Could you check a few things on this drawing? It's one solid part, dimensions in mm from its lowest x, y, z. A direction names the side the tool comes from. Give positions to 0.01 mm unless a question says otherwise; leave off trailing zeros. Order: outer loops, then holes, each group sorted by start corner. A loop starts at its lowest first (then second) coordinate and runs counter-clockwise, first axis right, second up.
Item 1: If we mould it in two halves opening along Z, with no side actions, what happens to the marked faces 1, 2, 3 and 4? For each: +Z half, -Z half, draft (parallel to the pull), parting line (faces both ways), or undercut.
Item 2: I want a section at A-A, the plane z = 14. Write out the boundary of the cut face in (x, y), then the cut area to 3 significant figures.
Item 3: I want a section at C-C, the plane y = 15. Write out the boundary of the cut face in (x, z), then the cut area to 3 significant figures.
Item 4: Which directions (+Z, -Z, +X, -X, +Y, -Y) give clear straight access to the entire face, cutting with the end or side of a thin tool? Please do the marked faces 5 and 6.
Item 5: I'm going to push flat-ended pins straight in: pin 1 Ø6 at (x, y) = (50.5, 20.5) entering from -Z; pin 2 Ø5 at (x, z) = (73, 67) entering from +Y. Where does each tip first touch, or does it pass through?
Item 6: If I drill on line 1 along X through (y, z) = (25, 46); line 2 along Z through (x, y) = (40.5, 5.5), over which ranges is the centre line in solid material (lowest first)?
Item 7: I want a section at B-B, the plane x = 15. Write out the boundary of the cut face in (y, z), then the cut area to 3 significant figures.
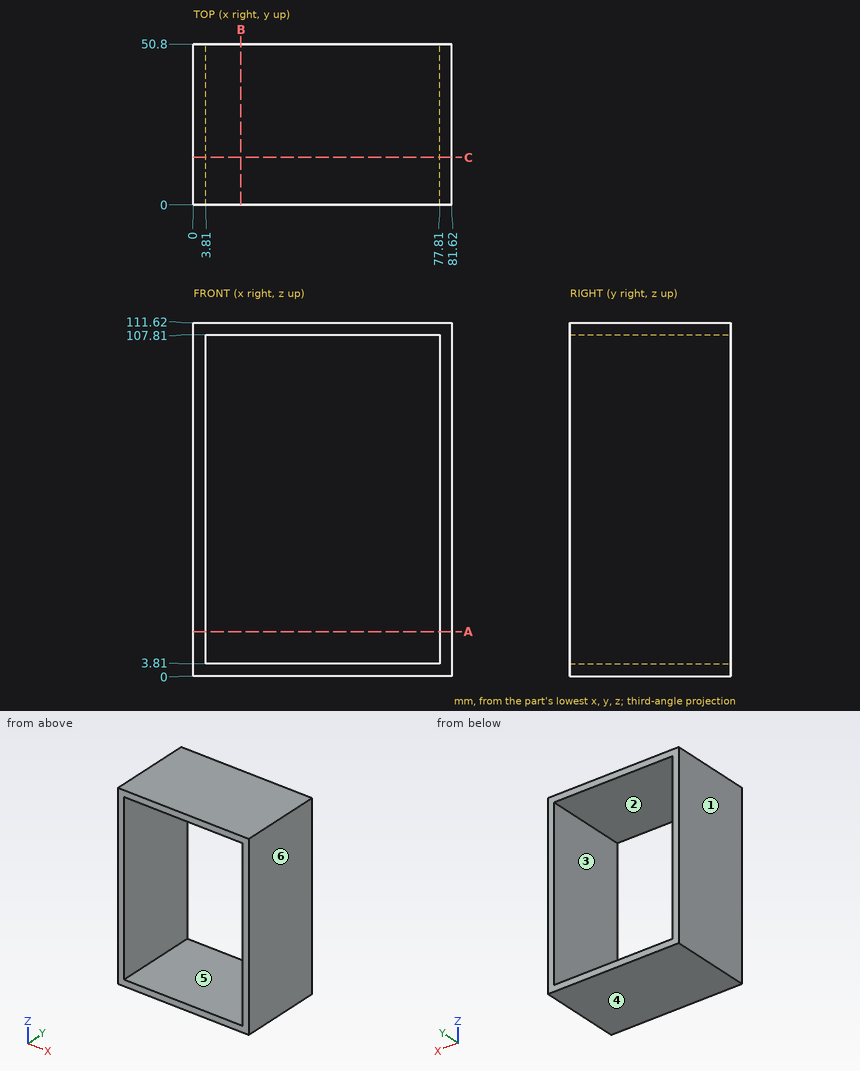
Results list:
1. face 1: draft
1. face 2: undercut
1. face 3: undercut
1. face 4: -Z half
2. outline: (0, 0) - (3.81, 0) - (3.81, 50.8) - (0, 50.8) - close; (77.81, 0) - (81.62, 0) - (81.62, 50.8) - (77.81, 50.8) - close
2. area: 387 mm2
3. outline: (0, 0) - (81.62, 0) - (81.62, 111.62) - (0, 111.62) - close; hole (3.81, 3.81) - (77.81, 3.81) - (77.81, 107.81) - (3.81, 107.81) - close
3. area: 1,410 mm2
4. face 5: +Y, -Y
4. face 6: +Z, -Z, +X, +Y, -Y
5. pin 1: stops at z = 0
5. pin 2: passes through
6. line 1: x = 0 to 3.81, 77.81 to 81.62
6. line 2: z = 0 to 3.81, 107.81 to 111.62
7. outline: (0, 0) - (50.8, 0) - (50.8, 3.81) - (0, 3.81) - close; (0, 107.81) - (50.8, 107.81) - (50.8, 111.62) - (0, 111.62) - close
7. area: 387 mm2
